from build123d import *

# Parameters (mm, degrees)
ESBO_O1_R                  = 1.5
RESSALTO_EXTRUS_O3_DEPTH   = 6.2
RESSALTO_EXTRUS_O3_2_DEPTH = 6.2
ESBO_O1_7_W                = 44.78884621
ESBO_O1_7_H                = 54.813199192
RESSALTO_EXTRUS_O4_DEPTH   = 3.2


with BuildPart() as part:
    # Esbo_o1 → Ressalto-extrus_o3 (new body)
    with BuildSketch(Plane.XY):
        Polygon((4.764517869, 71.802052111), (4.764517869, 82.395452515), (-35.446635921, 82.395452515), (-35.446635921, 91.395452515), (4.764517869, 91.395452515), (4.764517869, 101.988852919), (49.553364079, 101.988852919), (49.553364079, 71.802052111), align=None)
        with Locations(Location((30.053364079, 86.895452515, 0), (0, 0, 180))):
            Circle(ESBO_O1_R, mode=Mode.SUBTRACT)
        with Locations(Location((15.053364079, 96.395452515, 0), (0, 0, 180))):
            Circle(ESBO_O1_R, mode=Mode.SUBTRACT)
        with Locations(Location((15.053364079, 77.395452515, 0), (0, 0, 180))):
            Circle(ESBO_O1_R, mode=Mode.SUBTRACT)
        with Locations(Location((-26.946635921, 86.895452515, 0), (0, 0, 180))):
            Circle(ESBO_O1_R, mode=Mode.SUBTRACT)
    extrude(amount=RESSALTO_EXTRUS_O3_DEPTH)



with BuildPart() as body_2:
    # Esbo_o1 → Ressalto-extrus_o3 2 (new body)
    with BuildSketch(Plane.XY):
        Polygon((-35.446635921, 6.395452515), (-35.446635921, -2.604547485), (4.764517869, -2.604547485), (4.764517869, -13.197947889), (49.553364079, -13.197947889), (49.553364079, 16.988852919), (4.764517869, 16.988852919), (4.764517869, 6.395452515), align=None)
        with Locations(Location((15.053364079, -7.604547485, 0), (0, 0, 180))):
            Circle(ESBO_O1_R, mode=Mode.SUBTRACT)
        with Locations(Location((15.053364079, 11.395452515, 0), (0, 0, 180))):
            Circle(ESBO_O1_R, mode=Mode.SUBTRACT)
        with Locations(Location((30.053364079, 1.895452515, 0), (0, 0, 180))):
            Circle(ESBO_O1_R, mode=Mode.SUBTRACT)
        with Locations(Location((-26.946635921, 1.895452515, 0), (0, 0, 180))):
            Circle(ESBO_O1_R, mode=Mode.SUBTRACT)
    extrude(amount=RESSALTO_EXTRUS_O3_2_DEPTH)


with BuildPart() as part_1:
    add(part.part)

    add(body_2.part)  # Ressalto-extrus_o4 merges body 2
    # Esbo_o1_7 → Ressalto-extrus_o4 (add)
    with BuildSketch(Plane.XY):
        with Locations((27.158940974, 44.395452515)):
            Rectangle(ESBO_O1_7_W, ESBO_O1_7_H)
    extrude(amount=RESSALTO_EXTRUS_O4_DEPTH)


solid = part_1.part
CAD build for the part. Positions are in the model's coordinates, mm. A direction names the side the tool comes from. Coordinates: 2 decimals unless noted, no trailing zeros. Write each loop counter-clockwise with the first axis right and the second up, starting at its lowest first coordinate (ties: lowest second). Pieces come first, ordered by that corner, then holes. Notation, with made-up numbers: M -26.5,83.5 L 25.5,83.5 A32 ccw 25.5,109.5 Z; hole C 45.25,74 d5. An arc over 180 degrees is marked long. Return JSON: item names as keys, results as strings.
Item 1: Slice it at B-B, the plane z = 4.75. State how many separate pieces and enclosed holes the cut face has, and give its area (3 significant figures).
Findings below:
{"separate pieces": "2", "enclosed holes": "8", "area": "3,370 mm2"}
Item 2: Which spindle directions (+Z, -Z, +X, -X, +Y, -Y) get a long thin tool onto all of the face, cutting with end or side? Do faces 1 (the flat face through (4.765, -8, 3)), 2 (the flat face through (-16, 91.395, 3)), 3 (the flat face through (4.765, 44, 2)), 4 (the flat face through (27, 16.989, 5)). Say none if no direction does.
Findings below:
{"face 1": "+Z, -Z, -X, -Y", "face 2": "+Z, -Z, -X, +Y", "face 3": "+Z, -Z, -X", "face 4": "+Z, +X, -X"}
Item 3: Two-plate mould, pull along Y, no slides. Class faces 5 (the flat face through (27, 101.989, 3)), 6 (the flat face through (27, -13.198, 3)), 7 (the cylindrical face through (14.361, 78.726, 3.057)): +Y half, -Y half, draft (parallel to the pull), parting line (faces both ways), or undercut.
Findings below:
{"face 5": "+Y half", "face 6": "-Y half", "face 7": "undercut"}
Item 4: Probe line 1 (Y direction, x = 26, z = 5.5); line 2 (Y direction, x = 3, z = 2.25); line 3 (Y direction, x = -26, z = 6). List the from-to ranges inside material, lowest first. Write a range as from..to.
Findings below:
{"line 1": "y = -13.2..16.99, 71.8..101.99", "line 2": "y = -2.6..6.4, 82.4..91.4", "line 3": "y = -2.6..0.73, 3.06..6.4, 82.4..85.73, 88.06..91.4"}
Item 5: Slice it at A-A, the plane x = -15. Write the cut outline in (y, z).
Findings below:
{"outline": "M -2.6,0 L 6.4,0 L 6.4,6.2 L -2.6,6.2 Z; M 82.4,0 L 91.4,0 L 91.4,6.2 L 82.4,6.2 Z"}
Item 6: Drop flat-ended pins along their axis: pin 1 Ø2.5 at (x, y) = (15.05, -7.6) entering from -Z; pin 2 Ø3 at (y, z) = (48, 4) entering from -X. Give the stop position or say it passes through.
Findings below:
{"pin 1": "passes through", "pin 2": "stops at x = 4.76"}
Item 7: Slice it at C-C, the plane y = 27. Write the cut outline in (x, z), and give its area (3 significant figures).
Findings below:
{"outline": "M 4.76,0 L 49.55,0 L 49.55,3.2 L 4.76,3.2 Z", "area": "143 mm2"}
